Geometry: see drawing. Coordinates: mm, zero at the bounding-box minimum. A direction names the side the tool comes from. Round coordinates to 2 decimals unless told otherwise and drop trailing zeros. Write each loop counter-clockwise with the first axis right and the second up, starting at its lowest first coordinate (ties: lowest second). Pieces come first, ordered by that corner, then holes.
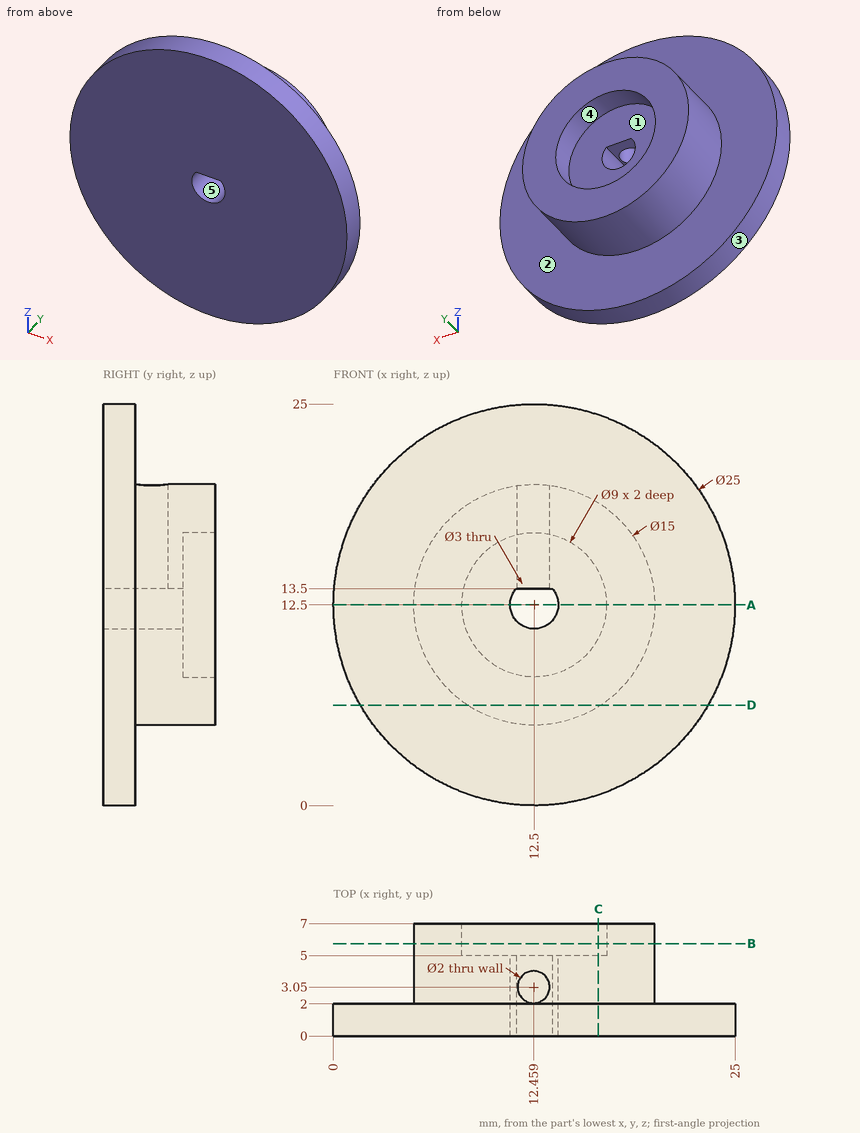
1) Section query B-B on y = 5.75. Return the cut outline in (x, z).
Taken from the geometry:
outline: circle Ø15 at (12.5, 12.5); hole circle Ø9 at (12.5, 12.5)
2) Section query A-A on z = 12.5. Return the cut outline in (x, y).
Taken from the geometry:
outline: (0, 0) - (11, 0) - (11, 5) - (8, 5) - (8, 7) - (5, 7) - (5, 2) - (0, 2) - close; (14, 0) - (25, 0) - (25, 2) - (20, 2) - (20, 7) - (17, 7) - (17, 5) - (14, 5) - close
3) Material intervals for line 1 (Z direction, x = 12.5, y = 6.2); line 2 (X direction, y = 3.5, z = 12.5), sorted ascending.
Taken from the geometry:
line 1: z = 5 to 8, 17 to 20
line 2: x = 5 to 11, 14 to 20
4) Reachability of the marked faces 4 and 5 from +Z, -Z, +X, -X, +Y, -Y: full face, straight path, thin tool, end or side. Return the list, or none.
Taken from the geometry:
face 4: +Y
face 5: +Y, -Y
5) Pull-direction query (X, two-part tool) for the marked faces 1, 2 and 3; classes: released by +X, released by -X, zero draft, split by the parting line, or undercut.
Taken from the geometry:
face 1: undercut
face 2: zero draft
face 3: split by the parting line
6) Contact query for flat-ended pins moving along their axis: P1, Ø4.5, axis at x = 13.5, z = 11, coming from the +Y side; P2, Ø2, axis at x = 5.5, y = 2, coming from the +Z side; P3, Ø1.1, axis at x = 12, y = 3, coming from the -Z side. Output: stop coordinate, or through.
Taken from the geometry:
P1: stops at y = 5
P2: stops at z = 23.47
P3: stops at z = 5
7) Section query C-C on x = 16.5. Return the cut outline in (y, z).
Taken from the geometry:
outline: (0, 0.66) - (2, 0.66) - (2, 6.16) - (7, 6.16) - (7, 10.44) - (5, 10.44) - (5, 14.56) - (7, 14.56) - (7, 18.84) - (2, 18.84) - (2, 24.34) - (0, 24.34) - close
8) Section query D-D on z = 6.25. Return the cut outline in (x, y) (1 decimal).
Taken from the geometry:
outline: (1.7, 0) - (23.3, 0) - (23.3, 2) - (16.6, 2) - (16.6, 7) - (8.4, 7) - (8.4, 2) - (1.7, 2) - close
